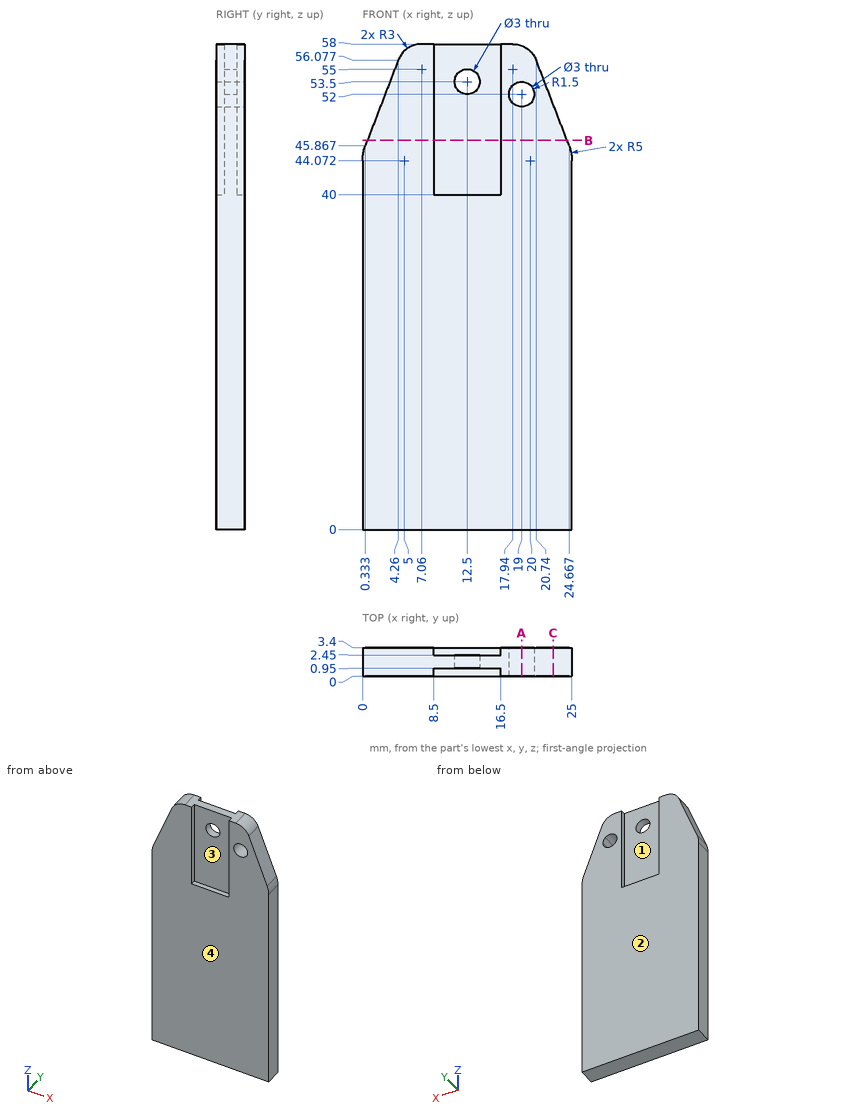
Geometry check sheet. Reference: drawing and pictorial views, mm from the part's lowest x, y, z. A direction names the side the tool comes from. Give positions to 0.01 mm unless a question says otherwise; leave off trailing zeros. Order: outer loops, then holes, each group sorted by start corner. A loop starts at its lowest first (then second) coordinate and runs counter-clockwise, first axis right, second up. Notation, with made-up numbers: M -0.75,86.25 L 9.25,86.25 A12 cw 9.25,91.25 Z; hole C -30,-9.5 d4. An arc over 180 degrees is marked long. Answer in a Markdown table with one row per item.
1) Cross-section at C-C, the plane x = 22.75. Enter the section's corners in (y, z), plus the area to 3 significant figures.
Filled sheet:
| item | result |
|---|---|
| outline | M 0,0 L 3.4,0 L 3.4,50.85 L 0,50.85 Z |
| area | 173 mm2 |
2) Gauge pin test, flat ends, axial feed: P1, Ø9, axis at x = 11.5, z = 52.5, coming from the +Y side; P2, Ø0.8, axis at y = 0.5, z = 50.5, coming from the -X side; P3, Ø0.8, axis at y = 0.5, z = 47.5, coming from the +X side; P4, Ø2.5, axis at x = 14, z = 49.5, coming from the -Y side. Record the tip position at first contact, or that the pin passes through.
Filled sheet:
| item | result |
|---|---|
| P1 | stops at y = 3.4 |
| P2 | stops at x = 1.96 |
| P3 | stops at x = 24.19 |
| P4 | stops at y = 0.95 |
3) Thickness scan on L1, parallel to Z at x = 12.5, y = 1.6; L2, parallel to Y at x = 9.5, z = 53.5; L3, parallel to Z at x = 19, y = 1.2 (1 decimal). Record the ranges inside material, lowest first. Write a range as [from, to].
Filled sheet:
| item | result |
|---|---|
| L1 | z = [0, 52], [55, 58] |
| L2 | y = [0.95, 2.45] |
| L3 | z = [0, 50.5], [53.5, 57.8] |
4) Cross-section at A-A, the plane x = 19. Enter the section's corners in (y, z).
Filled sheet:
| item | result |
|---|---|
| outline | M 0,0 L 3.4,0 L 3.4,50.5 L 0,50.5 Z; M 0,53.5 L 3.4,53.5 L 3.4,57.81 L 0,57.81 Z |
5) Access from +Z, -Z, +X, -X, +Y, -Y to the whole of each face (thin tool, end or side, straight path). Record for the marked faces 3 and 4.
Filled sheet:
| item | result |
|---|---|
| face 3 | +Z, -Y |
| face 4 | +Z, -Z, +X, -X, -Y |
6) Cross-section at B-B, the plane z = 46.5. Enter the section's corners in (x, y).
Filled sheet:
| item | result |
|---|---|
| outline | M 0.58,0 L 8.5,0 L 8.5,0.95 L 16.5,0.95 L 16.5,0 L 24.42,0 L 24.42,3.4 L 16.5,3.4 L 16.5,2.45 L 8.5,2.45 L 8.5,3.4 L 0.58,3.4 Z |
7) Release check for a two-part mould opening along X. For the marked faces 1 and 2 record: +X half, -X half, draft (parallel to the pull), parting line (faces both ways), or undercut.
Filled sheet:
| item | result |
|---|---|
| face 1 | undercut |
| face 2 | draft |
